Design review of the part built by this model. Coordinates are the model's own, in mm. Coordinates: 2 decimals unless noted, no trailing zeros. Loops run counter-clockwise (first coordinate to the right, second up) from the corner with the lowest first, then second, coordinate; pieces in that order, holes last. Notation, with made-up numbers: (20.25, -34.75) -> (79.25, -34.75) arc R18 ccw to (79.25, -15.75) -> close; hole circle Ø3 at (24, -3.75). An arc over 180 degrees is marked (long way). Answer in a Markdown table with one row per item.
```python
from build123d import *

# Parameters (mm, degrees)
SKETCH1_W            = 20.2
SKETCH1_H            = 10.2
BOSS_EXTRUDE1_DEPTH  = 10.6
SKETCH2_W            = 13
SKETCH2_H            = 10.2
SKETCH2_W_2          = 1.525
CUT_EXTRUDE1_DEPTH   = 0.5
SKETCH3_W            = 17.15
SKETCH3_H            = 9.76
CUT_EXTRUDE2_DEPTH   = 0.5
SKETCH4_W            = 0.48
SKETCH4_H            = 0.27
BOSS_EXTRUDE2_DEPTH  = 3.5
FILLET1_R            = 0.06
FILLET1_OF_MIRROR1_R = 0.06
FILLET2_R            = 0.05


with BuildPart() as part:
    # Sketch1 → Boss-Extrude1 (new body)
    with BuildSketch(Plane.XY):
        Rectangle(SKETCH1_W, SKETCH1_H)
    extrude(amount=BOSS_EXTRUDE1_DEPTH)

    # Sketch2 → Cut-Extrude1 (cut)
    with BuildSketch(Plane(origin=(0, 0, 0), x_dir=(-1, 0, 0), z_dir=(0, 0, -1))):
        Rectangle(SKETCH2_W, SKETCH2_H)
        with Locations((-9.3375, 0)):
            Rectangle(SKETCH2_W_2, SKETCH2_H)
        with Locations((9.3375, 0)):
            Rectangle(SKETCH2_W_2, SKETCH2_H)
    extrude(amount=-CUT_EXTRUDE1_DEPTH, mode=Mode.SUBTRACT)

    # Sketch3 → Cut-Extrude2 (cut)
    with BuildSketch(Plane(origin=(0, 0, 0), x_dir=(-1, 0, 0), z_dir=(0, 0, -1))):
        Rectangle(SKETCH3_W, SKETCH3_H)
    extrude(amount=-CUT_EXTRUDE2_DEPTH, mode=Mode.SUBTRACT)

    # Sketch4 → Boss-Extrude2 (add)
    with BuildSketch(Plane(origin=(0, 0, 0.5), x_dir=(-1, 0, 0), z_dir=(0, 0, -1))):
        with Locations((8.9, -3.81)):
            Rectangle(SKETCH4_W, SKETCH4_H)
        with Locations((6.36, -3.81)):
            Rectangle(SKETCH4_W, SKETCH4_H)
        with Locations((1.28, -3.81)):
            Rectangle(SKETCH4_W, SKETCH4_H)
        with Locations((-3.8, -3.81)):
            Rectangle(SKETCH4_W, SKETCH4_H)
        with Locations((-8.88, -3.81)):
            Rectangle(SKETCH4_W, SKETCH4_H)
    boss_extrude2 = extrude(amount=BOSS_EXTRUDE2_DEPTH)

    # Fillet1
    fillet1_edges = [part.edges().sort_by_distance(p)[0] for p in [
        (-6.6, -3.675, -1.25),
        (-6.6, -3.945, -1.25),
        (-6.12, -3.945, -1.25),
        (-6.12, -3.675, -1.25),
        (-1.52, -3.675, -1.25),
        (-1.52, -3.945, -1.25),
        (-1.04, -3.945, -1.25),
        (-1.04, -3.675, -1.25),
        (3.56, -3.675, -1.25),
        (3.56, -3.945, -1.25),
        (4.04, -3.945, -1.25),
        (4.04, -3.675, -1.25),
        (8.64, -3.675, -1.25),
        (8.64, -3.945, -1.25),
        (9.12, -3.945, -1.25),
        (9.12, -3.675, -1.25),
        (-8.66, -3.945, -1.25),
        (-8.66, -3.675, -1.25),
        (-9.14, -3.675, -1.25),
        (-9.14, -3.945, -1.25),
    ]]
    fillet(fillet1_edges, radius=FILLET1_R)

    # Mirror1: Boss-Extrude2 across plane
    add(boss_extrude2.mirror(Plane.ZX))

    # Fillet1 of Mirror1
    fillet1_of_mirror1_edges = [part.edges().sort_by_distance(p)[0] for p in [
        (-6.6, 3.675, -1.25),
        (-6.6, 3.945, -1.25),
        (-6.12, 3.945, -1.25),
        (-6.12, 3.675, -1.25),
        (-1.52, 3.675, -1.25),
        (-1.52, 3.945, -1.25),
        (-1.04, 3.945, -1.25),
        (-1.04, 3.675, -1.25),
        (3.56, 3.675, -1.25),
        (3.56, 3.945, -1.25),
        (4.04, 3.945, -1.25),
        (4.04, 3.675, -1.25),
        (8.64, 3.675, -1.25),
        (8.64, 3.945, -1.25),
        (9.12, 3.945, -1.25),
        (9.12, 3.675, -1.25),
        (-8.66, 3.945, -1.25),
        (-8.66, 3.675, -1.25),
        (-9.14, 3.675, -1.25),
        (-9.14, 3.945, -1.25),
    ]]
    fillet(fillet1_of_mirror1_edges, radius=FILLET1_OF_MIRROR1_R)

    # Fillet2
    fillet2_edges = [part.edges().sort_by_distance(p)[0] for p in [
        (-10.1, 0, 10.6),
        (0, -5.1, 10.6),
        (10.1, 0, 10.6),
        (0, 5.1, 10.6),
        (10.1, -5.1, 5.55),
        (-10.1, -5.1, 5.55),
        (-10.1, 5.1, 5.55),
        (10.1, 5.1, 5.55),
    ]]
    fillet(fillet2_edges, radius=FILLET2_R)


solid = part.part
```
(1) Take a section at A-A on z = 0.25. Count the separate pieces of the cut face and the enclosed holes in it, and give its area (3 significant figures).
Evaluation:
| item | result |
|---|---|
| separate pieces | 14 |
| enclosed holes | 0 |
| area | 3.09 mm² |
(2) To check wall thickness, follow probe 1 along Z at (x, y) = (8.5, -1.5); probe 2 along Y at (x, z) = (7.25, 0.25). State the ranges of each line that lie inside material, in increasing order.
Evaluation:
| item | result |
|---|---|
| probe 1 | z = 0.5 to 10.6 |
| probe 2 | y = -5.1 to -4.88, 4.88 to 5.1 |
(3) Take a section at D-D on x = -5. Give the boundary of the cut face in (y, z).
Evaluation:
| item | result |
|---|---|
| outline | (-5.1, 0.5) -> (5.1, 0.5) -> (5.1, 10.55) arc R0.05 ccw to (5.05, 10.6) -> (-5.05, 10.6) arc R0.05 ccw to (-5.1, 10.55) -> close |
(4) Take a section at C-C on y = 3. Give the boundary of the cut face in (x, z).
Evaluation:
| item | result |
|---|---|
| outline | (-10.1, 0.5) -> (10.1, 0.5) -> (10.1, 10.55) arc R0.05 ccw to (10.05, 10.6) -> (-10.05, 10.6) arc R0.05 ccw to (-10.1, 10.55) -> close |
(5) Draft analysis for pull direction Y (two halves, no side actions). For faces 1 (the flat face through (10.1, 0, 5)), 2 (the flat face through (0, 0, 0.5)), 3 (the flat face through (0, 5.1, 5)), 4 (the flat face through (0, -5.1, 5)), state which applies: pulls with the +Y half, pulls with the -Y half, needs draft (parallel to the pull), parting line crosses it, or undercut.
Evaluation:
| item | result |
|---|---|
| face 1 | needs draft |
| face 2 | undercut |
| face 3 | pulls with the +Y half |
| face 4 | pulls with the -Y half |
(6) For pin 1 (2 mm diameter, centred on x = -1, z = -1.5, fed in from +Y) (3 decimals); pin 2 (4 mm diameter, centred on x = -4, y = 0, fed in from -Z), all flat-tipped, find the tip position at first contact; note any pin that passes through.
Evaluation:
| item | result |
|---|---|
| pin 1 | stops at y = 3.945 |
| pin 2 | stops at z = 0.5 |
(7) Take a section at B-B on x = 7. Give the boundary of the cut face in (y, z), and give its area (3 significant figures).
Evaluation:
| item | result |
|---|---|
| outline | (-5.1, 0) -> (-4.88, 0) -> (-4.88, 0.5) -> (4.88, 0.5) -> (4.88, 0) -> (5.1, 0) -> (5.1, 10.55) arc R0.05 ccw to (5.05, 10.6) -> (-5.05, 10.6) arc R0.05 ccw to (-5.1, 10.55) -> close |
| area | 103 mm² |
